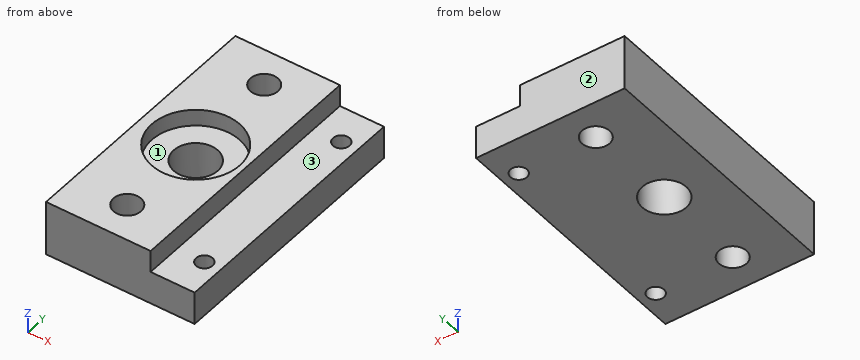
Autodesk Inventor part; units mm, degrees
ref_plane "YZ Plane" through (0, 0, 0) normal (1, 0, 0) x (0, 1, 0)
ref_plane "XZ Plane" through (0, 0, 0) normal (0, 1, 0) x (-1, 0, 0)
ref_plane "XY Plane" through (0, 0, 0) normal (0, 0, 1) x (1, 0, 0)
sketch "Sketch1" plane through (0, 0, 0) normal (0, 0, 1) x (1, 0, 0)
  line L0 (-13.5, -23.5) -> (13.5, -23.5)
  line L1 (13.5, -23.5) -> (13.5, 23.5)
  line L2 (13.5, 23.5) -> (-13.5, 23.5)
  line L3 (-13.5, 23.5) -> (-13.5, -23.5)
  line L4 (-13.5, -23.5) -> (13.5, 23.5) construction
  line L5 (13.5, -23.5) -> (-13.5, 23.5) construction
  point P0 (0, 0)
  dimension "d0" = 27
  dimension "d1" = 47
extrude "Extrusion1" add sketch "Sketch1" along normal blind 10
sketch "Sketch2" plane through (0, 0, 10) normal (0, 0, 1) x (1, 0, 0)
  line L0 (13.5, -23.5) -> (13.5, 23.5)
  line L1 (13.5, 23.5) -> (10.5, 23.5)
  line L2 (13.5, 23.5) -> (-13.5, 23.5)
  line L3 (10.5, 23.5) -> (10.5, 17)
  line L4 (10.5, 17) -> (10.5, -17)
  circle A0 centre (10.5, -17) radius 1.5
  circle A1 centre (10.5, 17) radius 1.5
  line L5 (13.5, 23.5) -> (10.5, 23.5)
  line L6 (13.5, 23.5) -> (-3.5, 23.5)
  line L7 (-3.5, 23.5) -> (-3.5, 17)
  circle A2 centre (-3.5, 17) radius 2.5
  line L8 (-3.5, 23.5) -> (-3.5, 0)
  circle A3 centre (-3.5, 0) radius 4
  line L9 (-3.5, 0) -> (-3.5, -15.5)
  line L10 (-3.5, -15.5) -> (-3.5, -17)
  circle A4 centre (-3.5, -17) radius 2.5
  point P0 (0, 0)
  dimension "d4" = 3
  dimension "d5" = 6.5
  dimension "d6" = 34
  dimension "d7" = 3
  dimension "d8" = 3
  dimension "d9" = 17
  dimension "d10" = 6.5
  dimension "d11" = 5
  dimension "d12" = 8
  dimension "d13" = 5
extrude "Extrusion2" cut sketch "Sketch2" against normal through all
sketch "Sketch3" plane through (0, 0, 10) normal (0, 0, 1) x (1, 0, 0)
  circle A0 centre (-3.5, 0) radius 4
  circle A1 centre (-3.5, 0) radius 8
  point P0 (0, 0)
  dimension "d16" = 16
extrude "Extrusion3" cut sketch "Sketch3" against normal blind 3
sketch "Sketch4" plane through (0, 0, 10) normal (0, 0, 1) x (1, 0, 0)
  line L0 (13.5, -23.5) -> (13.5, 23.5)
  line L1 (-13.5, -23.5) -> (13.5, -23.5)
  line L2 (13.5, 23.5) -> (5.5, 23.5)
  line L3 (5.5, 23.5) -> (5.5, -23.5)
  line L4 (5.5, -23.5) -> (13.5, -23.5)
  line L5 (13.5, -23.5) -> (13.5, 23.5)
  point P0 (0, 0)
  dimension "d19" = 8
extrude "Extrusion4" cut sketch "Sketch4" against normal blind 4
thread "Thread1"
thread "Thread2"
properties part number "Szorítólap"
Source: CAD feature listing. Evaluate the final solid. Frame: model axes, mm. Face numbers are marked on the shaded views. Coordinates: 2 decimals unless noted, no trailing zeros. Order: outer loops, then holes, each group sorted by start corner. A loop starts at its lowest first (then second) coordinate and runs counter-clockwise, first axis right, second up.
Item 1: First-contact query: P1, Ø12, axis at x = 6, y = -16, coming from the -Z side; P2, Ø5, axis at x = -3.5, y = 0, coming from the +Z side; P3, Ø2.5, axis at x = 8, y = -0.5, coming from the +Z side. Flat tips, straight axial feed; report the tip coordinate or a pass-through.
Output values:
P1: stops at z = 0
P2: passes through
P3: stops at z = 6
Item 2: Pull-direction query (Y, two-part tool) for the marked faces 1, 2 and 3; classes: pulls with the +Y half, pulls with the -Y half, needs draft (parallel to the pull), parting line crosses it, or undercut.
Output values:
face 1: undercut
face 2: pulls with the +Y half
face 3: needs draft
Item 3: Cut plane A-A (y = 0). Return loops of the section in (x, z), plus the area to 3 significant figures.
Output values:
outline: (-13.5, 0) - (-7.5, 0) - (-7.5, 7) - (-11.5, 7) - (-11.5, 10) - (-13.5, 10) - close; (0.5, 0) - (13.5, 0) - (13.5, 6) - (5.5, 6) - (5.5, 10) - (4.5, 10) - (4.5, 7) - (0.5, 7) - close
area: 134 mm2
Item 4: Cut plane C-C (z = 7.5). Return loops of the section in (x, y).
Output values:
outline: (-13.5, -23.5) - (5.5, -23.5) - (5.5, 23.5) - (-13.5, 23.5) - close; hole circle Ø16 at (-3.5, 0); hole circle Ø5 at (-3.5, -17); hole circle Ø5 at (-3.5, 17)
Item 5: Cut plane D-D (x = 10.5). Return loops of the section in (y, z).
Output values:
outline: (-23.5, 0) - (-18.5, 0) - (-18.5, 6) - (-23.5, 6) - close; (-15.5, 0) - (15.5, 0) - (15.5, 6) - (-15.5, 6) - close; (18.5, 0) - (23.5, 0) - (23.5, 6) - (18.5, 6) - close
Item 6: Material intervals for line 1 (Y direction, x = -3.5, z = 4.5); line 2 (Y direction, x = 10.5, z = 3.3); line 3 (Y direction, x = -1.75, z = 0.5), sorted ascending.
Output values:
line 1: y = -23.5 to -19.5, -14.5 to -4, 4 to 14.5, 19.5 to 23.5
line 2: y = -23.5 to -18.5, -15.5 to 15.5, 18.5 to 23.5
line 3: y = -23.5 to -18.79, -15.21 to -3.6, 3.6 to 15.21, 18.79 to 23.5
Item 7: Cut plane B-B (x = -3.5). Return loops of the section in (y, z).
Output values:
outline: (-23.5, 0) - (-19.5, 0) - (-19.5, 10) - (-23.5, 10) - close; (-14.5, 0) - (-4, 0) - (-4, 7) - (-8, 7) - (-8, 10) - (-14.5, 10) - close; (4, 0) - (14.5, 0) - (14.5, 10) - (8, 10) - (8, 7) - (4, 7) - close; (19.5, 0) - (23.5, 0) - (23.5, 10) - (19.5, 10) - close
